Can you work these out from the model? Positions are in its coordinate system, mm. A direction names the side the tool comes from. Coordinates: 2 decimals unless noted, no trailing zeros. Order: outer loops, then holes, each group sorted by start corner. A loop starts at its lowest first (then second) coordinate and runs counter-clockwise, first axis right, second up. Notation, with made-up numbers: (25, 66.25) -> (36, 66.25) arc R17 ccw to (36, 81.25) -> close; hole circle Ø8 at (67, 45). An arc over 180 degrees is marked (long way). Use a Markdown table: item, result. Add a question column.
1. Suppose I cut it at C-C, the plane y = 64.5. List the corners of the cut face in (x, z) for me.
2. Suppose I cut it at A-A, the plane x = -545.5. List the corners of the cut face in (y, z) for me.
3. For faces 1 (the flat face through (-472, 110, -831)), 2 (the flat face through (-545, 550, -658)), 3 (the flat face through (-575.513, 451, -824)), which set-ups out of +Z, -Z, +X, -X, +Y, -Y let a thin tool reach every point of the face, with its end or its side?
4. Suppose I cut it at B-B, the plane z = -773.5. List the corners of the cut face in (x, y) for me.
5. For pin 1 Ø5 at (x, z) = (-580, -544) entering from -Y; pin 2 Ø15 at (x, z) = (-452, -838.5) entering from +Y, each with a flat end and sliding along its axis, tell me the tip position at first contact or that it passes through.
6. If I drill on line 1 along Z through (x, y) = (-555.5, 82.5); line 2 along X through (y, z) = (577, -805); line 3 along Y through (x, z) = (-450.5, -812.5), over which ranges is the centre line in solid material (lowest first)? Write a range as from..to.
Autodesk Inventor part; units mm, degrees
ref_plane "YZ Plane" through (0, 0, 0) normal (1, 0, 0) x (0, 1, 0)
ref_plane "XZ Plane" through (0, 0, 0) normal (0, 1, 0) x (-1, 0, 0)
ref_plane "XY Plane" through (0, 0, 0) normal (0, 0, 1) x (1, 0, 0)
ref_plane "Work Plane1" through (0, 0, -806) normal (0, 0, -1) x (-1, 0, 0)
sketch "Sketch1" plane through (0, 0, -806) normal (0, 0, -1) x (-1, 0, 0)
  line L0 (428.0132, 10) -> (663.0132, 10)
  line L1 (663.0132, 10) -> (663.0132, 110)
  line L2 (663.0132, 110) -> (428.0132, 110)
  line L3 (428.0132, 110) -> (428.0132, 10)
  point P0 (0, 0)
extrude "Extrusion1" add sketch "Sketch1" along normal blind 50
sketch "Sketch2" plane through (-663.0132, 110, -806) normal (0, 1, 0) x (1, 0, 0)
  line L0 (117.5, 50) -> (147.5, 50)
  line L1 (0, 0) -> (235, 0)
  line L2 (147.5, 50) -> (87.5, 50)
  line L3 (87.5, 50) -> (87.5, 0)
  line L4 (87.5, 0) -> (147.5, 0)
  line L5 (147.5, 0) -> (147.5, 50)
  point P0 (663.0132, -806)
  dimension "d4" = 60
extrude "Extrusion2" add sketch "Sketch2" along normal blind 500
sketch "Sketch3" plane through (0, 0, -806) normal (0, 0, 1) x (1, 0, 0)
  line L0 (-663.0132, 10) -> (-663.0132, 110)
  line L1 (-428.0132, 10) -> (-663.0132, 10)
  line L2 (-428.0132, 110) -> (-428.0132, 10)
  line L3 (-515.5132, 110) -> (-428.0132, 110)
  line L4 (-515.5132, 110) -> (-515.5132, 610)
  line L5 (-575.5132, 610) -> (-515.5132, 610)
  line L6 (-575.5132, 110) -> (-575.5132, 610)
  line L7 (-663.0132, 110) -> (-575.5132, 110)
  line L8 (-575.5132, 110) -> (-575.5132, 610)
  line L9 (-515.5132, 110) -> (-515.5132, 610)
  line L10 (-575.5132, 610) -> (-515.5132, 610)
  line L11 (-515.5132, 610) -> (-515.5132, 550)
  line L12 (-515.5132, 550) -> (-575.5132, 550)
  line L13 (-575.5132, 550) -> (-575.5132, 610)
  point P0 (0, 0)
  dimension "d7" = 60
extrude "Extrusion3" add sketch "Sketch3" along normal blind 300 contours L6 L5 L4 L12
sketch "Sketch4" plane through (-663.0132, 610, -806) normal (0, 1, 0) x (1, 0, 0)
  point P0 (663.0132, -806)
Worked out:
| question | item | result |
|---|---|---|
| 1 | outline | (-663.01, -856) -> (-428.01, -856) -> (-428.01, -806) -> (-663.01, -806) -> close |
| 2 | outline | (10, -856) -> (610, -856) -> (610, -506) -> (550, -506) -> (550, -806) -> (10, -806) -> close |
| 3 | face 1 | +Z, -Z, +X, +Y |
| 3 | face 2 | +Z, +X, -X, -Y |
| 3 | face 3 | +Z, -Z, -X, +Y |
| 4 | outline | (-575.51, 550) -> (-515.51, 550) -> (-515.51, 610) -> (-575.51, 610) -> close |
| 5 | pin 1 | passes through |
| 5 | pin 2 | stops at y = 110 |
| 6 | line 1 | z = -856..-806 |
| 6 | line 2 | x = -575.51..-515.51 |
| 6 | line 3 | y = 10..110 |
